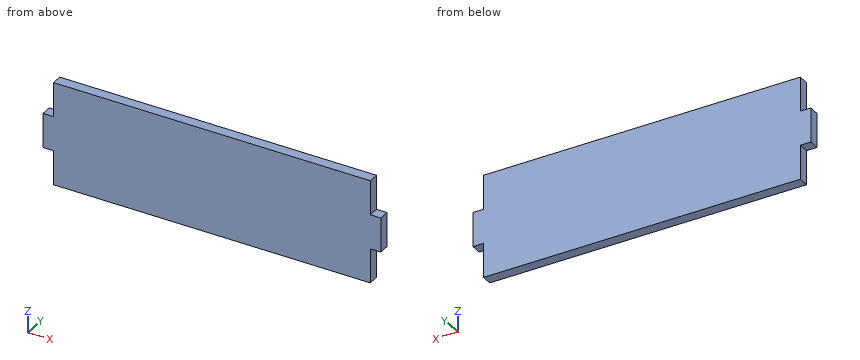
```python
from build123d import *

# Parameters (mm, degrees)
SKETCH1_W           = 193
SKETCH1_H           = 59
BOSS_EXTRUDE1_DEPTH = 6
SKETCH1_3_W         = 6
SKETCH1_3_H         = 19.666666667
CUT_EXTRUDE1_DEPTH  = 7


with BuildPart() as part:
    # Sketch1 → Boss-Extrude1 (new body)
    with BuildSketch(Plane(origin=(0, 0, 0), x_dir=(1, 0, 0), z_dir=(0, 1, 0))):
        Rectangle(SKETCH1_W, SKETCH1_H)
    extrude(amount=BOSS_EXTRUDE1_DEPTH)

    # Sketch1<3> → Cut-Extrude1 (cut, through all)
    with BuildSketch(Plane(origin=(0, 0, 0), x_dir=(1, 0, 0), z_dir=(0, 1, 0))):
        with Locations((-93.5, -19.666666667)):
            Rectangle(SKETCH1_3_W, SKETCH1_3_H)
        with Locations((-93.5, 19.666666667)):
            Rectangle(SKETCH1_3_W, SKETCH1_3_H)
    cut_extrude1 = extrude(amount=CUT_EXTRUDE1_DEPTH, mode=Mode.SUBTRACT)

    # Mirror1: Cut-Extrude1 across plane
    add(cut_extrude1.mirror(Plane(origin=(0, 0, 0), x_dir=(0, 0, 1), z_dir=(1, 0, 0))), mode=Mode.SUBTRACT)


solid = part.part
```
Geometry check sheet. Reference: the model listing, model coordinates, mm. Give positions to 0.01 mm unless a question says otherwise; leave off trailing zeros. Write each loop counter-clockwise with the first axis right and the second up, starting at its lowest first coordinate (ties: lowest second). Pieces come first, ordered by that corner, then holes.
1) Gauge pin test, flat ends, axial feed: pin 1 (1.8 mm diameter, centred on y = 2.5, z = 21, fed in from +X); pin 2 (3 mm diameter, centred on y = 2.5, z = 14.5, fed in from -X); pin 3 (1.8 mm diameter, centred on x = 94.5, y = 3.5, fed in from -Z). Record the tip position at first contact, or that the pin passes through.
2) Material ranges on L1, parallel to X at y = 1.5, z = 12, recorded low to high.
3) Section check A-A, the plane y = 5.1. Record the boundary of the cut face in (x, z).
4) Section check B-B, the plane z = 23.5. Record the boundary of the cut face in (x, y), and give its area (3 significant figures).
Computed:
1. pin 1: stops at x = 90.5
1. pin 2: stops at x = -90.5
1. pin 3: stops at z = -9.83
2. L1: x = -90.5 to 90.5
3. outline: (-96.5, -9.83) - (-90.5, -9.83) - (-90.5, -29.5) - (90.5, -29.5) - (90.5, -9.83) - (96.5, -9.83) - (96.5, 9.83) - (90.5, 9.83) - (90.5, 29.5) - (-90.5, 29.5) - (-90.5, 9.83) - (-96.5, 9.83) - close
4. outline: (-90.5, 0) - (90.5, 0) - (90.5, 6) - (-90.5, 6) - close
4. area: 1,090 mm2
